```python
from build123d import *

# Parameters (mm, degrees)
SKETCH1_W               = 152.4
SKETCH1_H               = 304.8
SKETCH1_W_2             = 101.6
SKETCH1_H_2             = 254
BOSS_EXTRUDE1_DEPTH     = 304.8
SKETCH2_W               = 101.6
SKETCH2_H               = 254
CUT_EXTRUDE1_DEPTH      = 304.8
SKETCH5_W               = 254
SKETCH5_H               = 254
CUT_EXTRUDE2_DEPTH      = 374.3022368
BOSS_EXTRUDE2_START     = -304.8
BOSS_EXTRUDE2_OUTLINE_W = 101.6
BOSS_EXTRUDE2_OUTLINE_H = 25.4
BOSS_EXTRUDE2_DEPTH     = 304.8
SKETCH6_W               = 101.6
SKETCH6_H               = 25.4
BOSS_EXTRUDE3_DEPTH     = 152.4
SKETCH7_W               = 30.48
SKETCH7_H               = 58.42
CUT_EXTRUDE3_DEPTH      = 25.654
SKETCH8_W               = 101.6
SKETCH8_H               = 50.8
BOSS_EXTRUDE4_DEPTH     = 25.4


# Read off the part's stored shape, not the designer's step: Boss-Extrude2
with BuildPart() as part:
    # Sketch1 → Boss-Extrude1 (new body)
    with BuildSketch(Plane(origin=(0, 0, 0), x_dir=(1, 0, 0), z_dir=(0, 1, 0))):
        Rectangle(SKETCH1_W, SKETCH1_H)
        Rectangle(SKETCH1_W_2, SKETCH1_H_2, mode=Mode.SUBTRACT)
    extrude(amount=BOSS_EXTRUDE1_DEPTH)

    # Sketch2 → Cut-Extrude1 (cut)
    with BuildSketch(Plane.XY.offset(152.4)):
        with Locations((0, 152.4)):
            Rectangle(SKETCH2_W, SKETCH2_H)
    extrude(amount=-CUT_EXTRUDE1_DEPTH, mode=Mode.SUBTRACT)

    # Sketch5 → Cut-Extrude2 (cut, through all)
    with BuildSketch(Plane(origin=(76.2, 0, 0), x_dir=(0, 0, -1), z_dir=(1, 0, 0))):
        with Locations((0, 152.4)):
            Rectangle(SKETCH5_W, SKETCH5_H)
    extrude(amount=-CUT_EXTRUDE2_DEPTH, mode=Mode.SUBTRACT)

    # Boss-Extrude2 outline → Boss-Extrude2 (add)
    with BuildSketch(Plane.XZ.offset(BOSS_EXTRUDE2_START)):
        with Locations((0, -12.7)):
            Rectangle(BOSS_EXTRUDE2_OUTLINE_W, BOSS_EXTRUDE2_OUTLINE_H)
    extrude(amount=BOSS_EXTRUDE2_DEPTH)

    # Sketch6 → Boss-Extrude3 (add)
    with BuildSketch(Plane.XY):
        with Locations((0, 215.9)):
            Rectangle(SKETCH6_W, SKETCH6_H)
    extrude(amount=BOSS_EXTRUDE3_DEPTH)

    # Sketch7 → Cut-Extrude3 (cut)
    with BuildSketch(Plane.XY):
        with Locations((0, 257.81)):
            Rectangle(SKETCH7_W, SKETCH7_H)
    extrude(amount=-CUT_EXTRUDE3_DEPTH, mode=Mode.SUBTRACT)

    # Sketch8 → Boss-Extrude4 (add)
    with BuildSketch(Plane.XY.offset(152.4)):
        with Locations((0, 254)):
            Rectangle(SKETCH8_W, SKETCH8_H)
    extrude(amount=-BOSS_EXTRUDE4_DEPTH)


solid = part.part
```
CAD build for the part. Positions are in the model's coordinates, mm. A direction names the side the tool comes from. Coordinates: 2 decimals unless noted, no trailing zeros. Order: outer loops, then holes, each group sorted by start corner. A loop starts at its lowest first (then second) coordinate and runs counter-clockwise, first axis right, second up. Notation, with made-up numbers: M 70.25,-1.5 L 94.25,-1.5 A12 ccw 94.25,15.5 Z; hole C 55,9.5 d1. An arc over 180 degrees is marked long. Write each question's results on one line, items separated by ' | '. Start each with the question number.
Q1. Which spindle directions (+Z, -Z, +X, -X, +Y, -Y) get a long thin tool onto all of the face, cutting with end or side? Do faces 4 (the flat face through (-50.8, 180, -0.4)), 5 (the flat face through (50.8, 292, 64)), 6 (the flat face through (-1, 13, 127)), 7 (the flat face through (-50.8, 151, -140)). Say none if no direction does.
Q2. Drill centre lines: probe 1 along Z at (x, y) = (-32, 293); probe 2 along X at (y, z) = (285, -121); probe 3 along Y at (x, z) = (53, 114). Where is each one in solid material? Low to high. Write a range as from..to.
Q3. Cut at A-A (z = 101). List the corners of the cut face in (x, y), then the cut area to 3 significant figures.
Q4. Cut at B-B (x = 32). List the corners of the cut face in (y, z), then the cut area to 3 significant figures.
Q5. Cut at D-D (z = -73.5). List the corners of the cut face in (x, y).
Q6. Pull direction Z, two halves, no side cores. Call faces 1 (the flat face through (-63, 151, -127)), 2 (the flat face through (-50.8, 113, 140)), 3 (the flat face through (-52, 188, 152.4)): +Z half, -Z half, draft (parallel to the pull), parting line (faces both ways), or undercut.
Q7. Flat gauge pins, fed straight in: P1, Ø1.5, axis at x = 5, y = 274, coming from the -Z side; P2, Ø2, axis at x = 44, y = 178, coming from the +Z side; P3, Ø12, axis at y = 248, z = 9, coming from the -X side; P4, Ø6, axis at x = -33, y = 124.5, coming from the -Z side. Where does each tip first touch, or does it go through?
Q8. Cut at C-C (y = 263). List the corners of the cut face in (x, z), then the cut area to 3 significant figures.
Found:
1) face 4: -X | face 5: +Y | face 6: -Y | face 7: -Z
2) probe 1: -152.4..-127, -25.4..0, 127..152.4 | probe 2: -76.2..-50.8, 50.8..76.2 | probe 3: 0..25.4, 279.4..304.8
3) outline: M -76.2,0 L -50.8,0 L -50.8,25.4 L -76.2,25.4 Z; M -76.2,279.4 L -50.8,279.4 L -50.8,304.8 L -76.2,304.8 Z; M -50.8,203.2 L 50.8,203.2 L 50.8,228.6 L -50.8,228.6 Z; M 50.8,0 L 76.2,0 L 76.2,25.4 L 50.8,25.4 Z; M 50.8,279.4 L 76.2,279.4 L 76.2,304.8 L 50.8,304.8 Z | area: 5,160 mm²
4) outline: M 0,-152.4 L 25.4,-152.4 L 25.4,-127 L 0,-127 Z; M 0,-25.4 L 304.8,-25.4 L 304.8,0 L 228.6,0 L 228.6,127 L 304.8,127 L 304.8,152.4 L 203.2,152.4 L 203.2,0 L 0,0 Z; M 0,127 L 25.4,127 L 25.4,152.4 L 0,152.4 Z; M 279.4,-152.4 L 304.8,-152.4 L 304.8,-127 L 279.4,-127 Z | area: 15,500 mm²
5) outline: M -76.2,0 L -50.8,0 L -50.8,25.4 L -76.2,25.4 Z; M -76.2,279.4 L -50.8,279.4 L -50.8,304.8 L -76.2,304.8 Z; M 50.8,0 L 76.2,0 L 76.2,25.4 L 50.8,25.4 Z; M 50.8,279.4 L 76.2,279.4 L 76.2,304.8 L 50.8,304.8 Z
6) face 1: undercut | face 2: draft | face 3: +Z half
7) P1: z = 127 | P2: z = 0 | P3: through | P4: z = -25.4
8) outline: M -76.2,-152.4 L -50.8,-152.4 L -50.8,-127 L -76.2,-127 Z; M -76.2,127 L 76.2,127 L 76.2,152.4 L -76.2,152.4 Z; M -50.8,-25.4 L -15.24,-25.4 L -15.24,0 L -50.8,0 Z; M 15.24,-25.4 L 50.8,-25.4 L 50.8,0 L 15.24,0 Z; M 50.8,-152.4 L 76.2,-152.4 L 76.2,-127 L 50.8,-127 Z | area: 6,970 mm²
